Can you work these out from the model? Positions are in its coordinate system, mm. A direction names the side the tool comes from. Coordinates: 2 decimals unless noted, no trailing zeros. Order: outer loops, then holes, each group sorted by start corner. A loop starts at its lowest first (then second) coordinate and runs counter-clockwise, first axis right, second up. Notation, with made-up numbers: M 8.5,-32.5 L 43.5,-32.5 A23 cw 43.5,-8.5 Z; hole C 56.5,-9 d9. An arc over 180 degrees is marked long. Answer as a JSON object with one key per item and string values.
from build123d import *

# Parameters (mm, degrees)
SKETCH1_W           = 54.6
SKETCH1_H           = 84
BOSS_EXTRUDE1_DEPTH = 8.15
SKETCH2_W           = 2
SKETCH2_H           = 84
CUT_EXTRUDE1_DEPTH  = 3.2
CHAMFER1_SIZE       = 0.1
BOSS_EXTRUDE2_DEPTH = 4.95
CUT_EXTRUDE4_DEPTH  = 4.95


with BuildPart() as part:
    # Sketch1 → Boss-Extrude1 (new body)
    with BuildSketch(Plane(origin=(0, 0, 0), x_dir=(1, 0, 0), z_dir=(0, 1, 0))):
        Rectangle(SKETCH1_W, SKETCH1_H)
    extrude(amount=BOSS_EXTRUDE1_DEPTH)

    # Sketch2 → Cut-Extrude1 (cut)
    with BuildSketch(Plane(origin=(0, 8.15, 0), x_dir=(1, 0, 0), z_dir=(0, 1, 0))):
        Rectangle(SKETCH2_W, SKETCH2_H)
    extrude(amount=-CUT_EXTRUDE1_DEPTH, mode=Mode.SUBTRACT)

    # Chamfer1
    chamfer1_edges = [part.edges().sort_by_distance(p)[0] for p in [
        (-27.3, 8.15, 0),
        (-14.15, 8.15, 42),
        (-14.15, 8.15, -42),
        (14.15, 8.15, 42),
        (1, 8.15, 0),
        (-1, 8.15, 0),
        (27.3, 8.15, 0),
        (14.15, 8.15, -42),
    ]]
    chamfer(chamfer1_edges, length=CHAMFER1_SIZE)

    # Sketch6 → Boss-Extrude2 (add)
    with BuildSketch(Plane(origin=(0, 0, 0), x_dir=(1, 0, 0), z_dir=(0, 1, 0))):
        with BuildLine():
            Line((-27.3, 26.3), (-27.3, 28.3))
            ThreePointArc((-27.3, 28.3), (-28.3, 27.3), (-27.3, 26.3))
        make_face()
        with BuildLine():
            Line((-21.3, -42), (-23.3, -42))
            ThreePointArc((-23.3, -42), (-22.3, -43), (-21.3, -42))
        make_face()
        with BuildLine():
            Line((-27.3, -28.3), (-27.3, -26.3))
            ThreePointArc((-27.3, -26.3), (-28.3, -27.3), (-27.3, -28.3))
        make_face()
        with BuildLine():
            Line((1, -42), (-1, -42))
            ThreePointArc((-1, -42), (0, -43), (1, -42))
        make_face()
        with BuildLine():
            Line((23.3, -42), (21.3, -42))
            ThreePointArc((21.3, -42), (22.3, -43), (23.3, -42))
        make_face()
    extrude(amount=BOSS_EXTRUDE2_DEPTH)

    # Sketch13 → Cut-Extrude4 (cut)
    with BuildSketch(Plane(origin=(0, 0, 0), x_dir=(1, 0, 0), z_dir=(0, 1, 0))):
        with BuildLine():
            Line((27.3, 28.3), (27.3, 26.3))
            ThreePointArc((27.3, 26.3), (26.3, 27.3), (27.3, 28.3))
        make_face()
        with BuildLine():
            Line((-23.3, 42), (-21.3, 42))
            ThreePointArc((-21.3, 42), (-22.3, 41), (-23.3, 42))
        make_face()
        with BuildLine():
            Line((27.3, -26.3), (27.3, -28.3))
            ThreePointArc((27.3, -28.3), (26.3, -27.3), (27.3, -26.3))
        make_face()
        with BuildLine():
            Line((-1, 42), (1, 42))
            ThreePointArc((1, 42), (0, 41), (-1, 42))
        make_face()
        with BuildLine():
            Line((21.3, 42), (23.3, 42))
            ThreePointArc((23.3, 42), (22.3, 41), (21.3, 42))
        make_face()
    extrude(amount=CUT_EXTRUDE4_DEPTH, mode=Mode.SUBTRACT)


solid = part.part
Item 1: I want a section at B-B, the plane z = -2.5. Write out the boundary of the cut face in (x, y).
Answers follow:
{"outline": "M -27.3,0 L 27.3,0 L 27.3,8.05 L 27.2,8.15 L 1.1,8.15 L 1,8.05 L 1,4.95 L -1,4.95 L -1,8.05 L -1.1,8.15 L -27.2,8.15 L -27.3,8.05 Z"}
Item 2: Please list where these lines run through material, in increasing order: line 1 (X direction, y = 5.25, z = -25); line 2 (Z direction, x = -19, y = 0.75); line 3 (X direction, y = 3.75, z = 31.5).
Answers follow:
{"line 1": "x = -27.3 to -1, 1 to 27.3", "line 2": "z = -42 to 42", "line 3": "x = -27.3 to 27.3"}
Item 3: Which directions (+Z, -Z, +X, -X, +Y, -Y) give clear straight access to the entire face, cutting with the end or side of a thin tool? Please do faces 1 (the flat face through (-1, 7, 1)), 2 (the cylindrical face through (-22.3, 2.4, -41)), 3 (the flat face through (-1, 0, 0)).
Answers follow:
{"face 1": "+Z, -Z, +Y", "face 2": "-Z, -Y", "face 3": "+Z, -Z, +X, -X, -Y"}
Item 4: If we mould it in two halves opening along Z, with no side actions, what happens to faces 4 (the cylindrical face through (0, 2, 43)), 5 (the cylindrical face through (-28.3, 2.4, 27.3)), 6 (the flat face through (0, 4.95, 0)), 7 (the cylindrical face through (26.3, 2.4, -27.3))? For each: pulls with the +Z half, pulls with the -Z half, needs draft (parallel to the pull), parting line crosses it, or undercut.
Answers follow:
{"face 4": "pulls with the +Z half", "face 5": "undercut", "face 6": "needs draft", "face 7": "undercut"}
Item 5: I want a section at A-A, the plane y = 3.5. Write out the boundary of the cut face in (x, z).
Answers follow:
{"outline": "M -27.3,-42 L -23.3,-42 A1 cw -21.3,-42 L -1,-42 A1 cw 1,-42 L 21.3,-42 A1 cw 23.3,-42 L 27.3,-42 L 27.3,-28.3 A1 cw 27.3,-26.3 L 27.3,26.3 A1 cw 27.3,28.3 L 27.3,42 L 23.3,42 A1 ccw 21.3,42 L 1,42 A1 ccw -1,42 L -21.3,42 A1 ccw -23.3,42 L -27.3,42 L -27.3,28.3 A1 ccw -27.3,26.3 L -27.3,-26.3 A1 ccw -27.3,-28.3 Z"}
Item 6: I want a section at C-C, the plane x = 0. Write out the boundary of the cut face in (y, z), plus the area to 3 significant figures.
Answers follow:
{"outline": "M 0,-41 L 4.95,-41 L 4.95,43 L 0,43 Z", "area": "416 mm^2"}
Item 7: I'm going to push flat-ended pins straight in: pin 1 (2.5 mm diameter, centred on y = 6, z = 15.5, fed in from -X); pin 2 (0.5 mm diameter, centred on x = 22.5, z = -41.5, fed in from -Y); pin 3 (0.5 mm diameter, centred on x = -27.5, z = 27.5, fed in from +Y). Where does each tip first touch, or does it pass through?
Answers follow:
{"pin 1": "stops at x = -27.3", "pin 2": "stops at y = 4.95", "pin 3": "stops at y = 8.1"}
